```python
from build123d import *

# Parameters (mm, degrees)
F0_W     = 38.1
F0_H     = 31.75
F1_DEPTH = 25.4
F3_DEPTH = 25.401


with BuildPart() as f1:
    # F0 (on Front) → F1 (new body)
    with BuildSketch(Plane.XZ):
        with Locations((-19.05, 15.875)):
            Rectangle(F0_W, F0_H)
    extrude(amount=F1_DEPTH)

    # F2 (on face) → F3 (cut, through all)
    with BuildSketch(Plane(origin=(0, 0, 0), x_dir=(-1, 0, 0), z_dir=(0, 1, 0))):
        Polygon((0, 31.75), (0, 11.58768), (12.7, 11.58768), (25.4, 31.75), align=None)
    extrude(amount=-F3_DEPTH, mode=Mode.SUBTRACT)


solid = f1.part
```
Verification items for the finished model (mm, model axes). A direction names the side the tool comes from. Round coordinates to 2 decimals unless told otherwise and drop trailing zeros. Order: outer loops, then holes, each group sorted by start corner. A loop starts at its lowest first (then second) coordinate and runs counter-clockwise, first axis right, second up.
1) Material ranges on line 1 (Z direction, x = -9, y = -16.5); line 2 (Z direction, x = -17, y = -9); line 3 (X direction, y = -9.25, z = 24.5), recorded low to high.
Geometry says:
line 1: z = 0 to 11.59
line 2: z = 0 to 18.41
line 3: x = -38.1 to -20.83
2) Tool access check on faces 4 (the flat face through (-6, -13, 11.588)), 5 (the flat face through (0, -13, 6)). Record the directions out of +Z, -Z, +X, -X, +Y, -Y that give a thin tool (end or side, any length) a straight path to the whole face; none if there is none.
Geometry says:
face 4: +Z, +X, +Y, -Y
face 5: +Z, -Z, +X, +Y, -Y
3) Depth check by flat-ended pin: pin 1 (1 mm diameter, centred on x = -21, y = -20, fed in from +Z); pin 2 (4 mm diameter, centred on x = -13.5, y = -12.5, fed in from +Z); pin 3 (1.5 mm diameter, centred on x = -15.5, y = -19.5, fed in from +Z). Enter the tip coordinate at first touch or a pass-through.
Geometry says:
pin 1: stops at z = 25.56
pin 2: stops at z = 16.03
pin 3: stops at z = 17.22
4) Cross-section at A-A, the plane y = -13. Record the cut outline in (x, z).
Geometry says:
outline: (-38.1, 0) - (0, 0) - (0, 11.59) - (-12.7, 11.59) - (-25.4, 31.75) - (-38.1, 31.75) - close
5) Cross-section at B-B, the plane x = -24.5. Record the cut outline in (y, z).
Geometry says:
outline: (-25.4, 0) - (0, 0) - (0, 30.32) - (-25.4, 30.32) - close
6) Draft check along Y on faces 1 (the flat face through (-24, -25.4, 13)), 2 (the flat face through (-24, 0, 13)), 3 (the flat face through (-38.1, -13, 16)). Enter one of: +Y half, -Y half, draft (parallel to the pull), parting line (faces both ways), or undercut.
Geometry says:
face 1: -Y half
face 2: +Y half
face 3: draft
7) Cross-section at C-C, the plane z = 17.5. Record the cut outline in (x, y), plus the area to 3 significant figures.
Geometry says:
outline: (-38.1, -25.4) - (-16.42, -25.4) - (-16.42, 0) - (-38.1, 0) - close
area: 551 mm2
